from build123d import *

# Parameters (mm, degrees)
BOSS_EXTRUDE1_DEPTH                     = 6.35
M5X0_8_TAPPED_HOLE1_D                   = 4.2
SKETCH4_W                               = 40
SKETCH4_H                               = 35
CUT_EXTRUDE1_DEPTH                      = 128.437523909
FILLET1_R                               = 5
CBORE_FOR_M5_HEX_HEAD_BOLT1_D           = 5.8
CBORE_FOR_M5_HEX_HEAD_BOLT1_CBORE_D     = 12.24
CBORE_FOR_M5_HEX_HEAD_BOLT1_CBORE_DEPTH = 3.58
FILLET2_R                               = 10
FILLET3_R                               = 2
CBORE_FOR_M3_SHCS1_D                    = 3.4
CBORE_FOR_M3_SHCS1_CBORE_D              = 6.5
CBORE_FOR_M3_SHCS1_CBORE_DEPTH          = 3


with BuildPart() as part:
    # Base plate → Boss-Extrude1 (new body)
    with BuildSketch(Plane(origin=(0, 0, 0), x_dir=(1, 0, 0), z_dir=(0, 1, 0))):
        Polygon((55, -55), (-55, -55), (-55, -17.5), (-90, -17.5), (-90, 17.5), (-55, 17.5), (-55, 55), (-17.5, 55), (-17.5, 90), (17.5, 90), (17.5, 55), (55, 55), (55, 17.5), (90, 17.5), (90, -17.5), (55, -17.5), align=None)
    extrude(amount=BOSS_EXTRUDE1_DEPTH)

    # M5x0.8 Tapped Hole1 (through all)
    with Locations(Plane(origin=(0, 0, 0), x_dir=(-1, 0, 0), z_dir=(0, -1, 0))):
        with Locations((-20, 15), (20, 15), (20, -5), (-20, -5), (-30, 15), (-30, -5), (30, 15), (30, -5)):
            Hole(M5X0_8_TAPPED_HOLE1_D / 2)

    # Sketch4 → Cut-Extrude1 (cut, through all)
    with BuildSketch(Plane(origin=(0, 6.35, 0), x_dir=(1, 0, 0), z_dir=(0, 1, 0))):
        with Locations((0, -37.5)):
            Rectangle(SKETCH4_W, SKETCH4_H)
    extrude(amount=-CUT_EXTRUDE1_DEPTH, mode=Mode.SUBTRACT)

    # Fillet1
    fillet1_edges = [part.edges().sort_by_distance(p)[0] for p in [
        (17.5, 3.175, -90),
        (17.5, 3.175, -55),
        (55, 3.175, -55),
        (55, 3.175, -17.5),
        (90, 3.175, -17.5),
        (90, 3.175, 17.5),
        (55, 3.175, 17.5),
        (55, 3.175, 55),
        (-55, 3.175, 55),
        (-55, 3.175, 17.5),
        (-90, 3.175, 17.5),
        (-90, 3.175, -17.5),
        (-55, 3.175, -17.5),
        (-55, 3.175, -55),
        (-17.5, 3.175, -55),
        (-17.5, 3.175, -90),
        (20, 3.175, 55),
        (-20, 3.175, 55),
    ]]
    fillet(fillet1_edges, radius=FILLET1_R)

    # CBORE for M5 Hex Head Bolt1 (through all)
    with Locations(Plane.XZ):
        with Locations((-45, 45), (-45, -45), (45, -45), (45, 45)):
            CounterBoreHole(CBORE_FOR_M5_HEX_HEAD_BOLT1_D / 2, CBORE_FOR_M5_HEX_HEAD_BOLT1_CBORE_D / 2, CBORE_FOR_M5_HEX_HEAD_BOLT1_CBORE_DEPTH)

    # Fillet2
    fillet2_edges = [part.edges().sort_by_distance(p)[0] for p in [
        (-20, 3.175, 20),
        (20, 3.175, 20),
    ]]
    fillet(fillet2_edges, radius=FILLET2_R)

    # Fillet3
    # the kernel refuses this fillet: 2 mm, written as the material it takes off along each edge
    with BuildSketch(Plane(origin=(20, 6.35, 30), x_dir=(0, -1, 0), z_dir=(0, 0, 1)), Plane(origin=(-20, 6.35, 55), x_dir=(0, -1, 0), z_dir=(0, 0, -1))) as fillet3_piece_1:
        with BuildLine():
            CenterArc((FILLET3_R, FILLET3_R), FILLET3_R, 180, 90)
            Line((0, FILLET3_R), (0, 0))
            Line((0, 0), (FILLET3_R, 0))
        make_face()
    extrude(amount=25, mode=Mode.SUBTRACT)
    with BuildSketch(Plane(origin=(-10, 6.35, 20), x_dir=(0, -1, 0), z_dir=(1, 0, 0))) as fillet3_piece_2:
        with BuildLine():
            CenterArc((FILLET3_R, FILLET3_R), FILLET3_R, 180, 90)
            Line((0, FILLET3_R), (0, 0))
            Line((0, 0), (FILLET3_R, 0))
        make_face()
    extrude(amount=20, mode=Mode.SUBTRACT)
    with BuildSketch(Plane(origin=(-20, 0, 30), x_dir=(-1, 0, 0), z_dir=(0, 0, 1)), Plane(origin=(20, 0, 55), x_dir=(1, 0, 0), z_dir=(0, 0, -1))) as fillet3_piece_3:
        with BuildLine():
            CenterArc((FILLET3_R, -FILLET3_R), FILLET3_R, 90, 90)
            Line((0, -FILLET3_R), (0, 0))
            Line((0, 0), (FILLET3_R, 0))
        make_face()
    extrude(amount=25, mode=Mode.SUBTRACT)
    with BuildSketch(Plane(origin=(10, 0, 20), x_dir=(0, 0, -1), z_dir=(-1, 0, 0))) as fillet3_piece_4:
        with BuildLine():
            CenterArc((FILLET3_R, -FILLET3_R), FILLET3_R, 90, 90)
            Line((0, -FILLET3_R), (0, 0))
            Line((0, 0), (FILLET3_R, 0))
        make_face()
    extrude(amount=20, mode=Mode.SUBTRACT)
    with BuildSketch(Plane(origin=(10, 0, 30), x_dir=(1, 0, 0), z_dir=(0, 0, 1))) as fillet3_piece_5:
        with BuildLine():
            CenterArc((10 + FILLET3_R, FILLET3_R), FILLET3_R, 180, 90)
            Line((10, FILLET3_R), (10, 0))
            Line((10, 0), (10 + FILLET3_R, 0))
        make_face()
    revolve(axis=Axis((10, 0, 30), (0, 1, 0)), revolution_arc=90, mode=Mode.SUBTRACT)
    with BuildSketch(Plane(origin=(-10, 0, 30), x_dir=(0, 0, -1), z_dir=(1, 0, 0))) as fillet3_piece_6:
        with BuildLine():
            CenterArc((10 + FILLET3_R, FILLET3_R), FILLET3_R, 180, 90)
            Line((10, FILLET3_R), (10, 0))
            Line((10, 0), (10 + FILLET3_R, 0))
        make_face()
    revolve(axis=Axis((-10, 0, 30), (0, 1, 0)), revolution_arc=90, mode=Mode.SUBTRACT)
    with BuildSketch(Plane(origin=(-10, 6.35, 30), x_dir=(0, 0, -1), z_dir=(1, 0, 0))) as fillet3_piece_7:
        with BuildLine():
            CenterArc((10 + FILLET3_R, -FILLET3_R), FILLET3_R, 90, 90)
            Line((10 + FILLET3_R, 0), (10, 0))
            Line((10, 0), (10, -FILLET3_R))
        make_face()
    revolve(axis=Axis((-10, 6.35, 30), (0, 1, 0)), revolution_arc=90, mode=Mode.SUBTRACT)
    with BuildSketch(Plane(origin=(10, 6.35, 30), x_dir=(1, 0, 0), z_dir=(0, 0, 1))) as fillet3_piece_8:
        with BuildLine():
            CenterArc((10 + FILLET3_R, -FILLET3_R), FILLET3_R, 90, 90)
            Line((10 + FILLET3_R, 0), (10, 0))
            Line((10, 0), (10, -FILLET3_R))
        make_face()
    revolve(axis=Axis((10, 6.35, 30), (0, 1, 0)), revolution_arc=90, mode=Mode.SUBTRACT)

    # CBORE for M3 SHCS1 (through all)
    with Locations(Plane(origin=(0, 0, 0), x_dir=(-1, 0, 0), z_dir=(0, -1, 0))):
        with Locations((10, 84), (-10, 84), (0, 60.3), (-84, 10), (-84, -10), (-60.3, 0), (84, -10), (84, 10), (60.3, 0)):
            CounterBoreHole(CBORE_FOR_M3_SHCS1_D / 2, CBORE_FOR_M3_SHCS1_CBORE_D / 2, CBORE_FOR_M3_SHCS1_CBORE_DEPTH)


solid = part.part
The listing builds one solid part. Answer for the finished solid, in the listing's coordinates (mm). A direction names the side the tool comes from. Coordinates: 2 decimals unless noted, no trailing zeros. Write each loop counter-clockwise with the first axis right and the second up, starting at its lowest first coordinate (ties: lowest second). Pieces come first, ordered by that corner, then holes. Notation, with made-up numbers: M 77.5,-3 L 118.5,-3 A20 cw 118.5,20 Z; hole C 57.25,28.5 d3. An arc over 180 degrees is marked long. Put each result on its own line as item: value. Start each with the question number.
1. A cutting plane is placed at B-B on y = 1. Count the separate pieces of the cut face and the enclosed holes in it, then the cut area to 3 significant figures.
2. Which of the six approach directions +Z, -Z, +X, -X, +Y, -Y give full straight-line access (tool end or side, diameter ignored) to faces 4 (the cylindrical face through (-80.753, 1.479, 9.857)), 5 (the cylindrical face through (-22, 3, 54)), 6 (the flat face through (-36, 3, -55))?
3. Consider line 1 (Z direction, x = -45, y = 1.75); line 2 (X direction, y = 2.35, z = -84); line 3 (Z direction, x = -84, y = 4.35). Determine where each line is inside the solid, lowest interval first. Write a range as from..to.
4. For a pull along X with two mould halves and no side action, classify faces 1 (the flat face through (-37, 3, 55)), 2 (the cylindrical face through (-56.43, 3.22, -19)), 3 (the cylindrical face through (-39.163, 1.765, -43.162)) as pulls with the +X half, pulls with the -X half, needs draft (parallel to the pull), parting line crosses it, or undercut.
5. Flat-ended cylindrical pins translate along their axes: P1, Ø3, axis at x = -9, z = -83.5, coming from the -Y side; P2, Ø3.5, axis at x = -45, z = 45, coming from the +Y side (3 decimals); P3, Ø2, axis at y = 4.5, z = -69, coming from the -X side; P4, Ø1.2, axis at y = 3, z = 39, coming from the +X side. Find the tip coordinate at first contact, or state that the pin passes through.
6. A cutting plane is placed at A-A on z = -45. Write down the section's boundary in (x, y), then the cut area to 3 significant figures.
Resolved:
1. separate pieces: 1
1. enclosed holes: 21
1. area: 13,500 mm2
2. face 4: -Y
2. face 5: +Z, +Y, -Y
2. face 6: -Z, -X, +Y, -Y
3. line 1: z = -55..-51.12, -38.88..38.88, 51.12..55
3. line 2: x = -17.5..-13.25, -6.75..6.75, 13.25..17.5
3. line 3: z = -17.5..-11.7, -8.3..8.3, 11.7..17.5
4. face 1: needs draft
4. face 2: pulls with the -X half
4. face 3: undercut
5. P1: stops at y = 3
5. P2: passes through
5. P3: stops at x = -17.5
5. P4: stops at x = 55
6. outline: M -55,0 L -51.12,0 L -51.12,3.58 L -47.9,3.58 L -47.9,6.35 L -55,6.35 Z; M -42.1,3.58 L -38.88,3.58 L -38.88,0 L 38.88,0 L 38.88,3.58 L 42.1,3.58 L 42.1,6.35 L -42.1,6.35 Z; M 47.9,3.58 L 51.12,3.58 L 51.12,0 L 55,0 L 55,6.35 L 47.9,6.35 Z
6. area: 579 mm2
